```python
from build123d import *

# Parameters (mm, degrees)
BOSS_EXTRUDE1_DEPTH = 10
SKETCH2_W           = 10
SKETCH2_H           = 3
BOSS_EXTRUDE2_DEPTH = 10
SKETCH3_R           = 1.5
CUT_EXTRUDE1_DEPTH  = 3
FILLET1_R           = 15
SKETCH4_R           = 1.5
BOSS_EXTRUDE3_DEPTH = 3
FILLET2_R           = 5


with BuildPart() as part:
    # Sketch1 → Boss-Extrude1 (new body)
    with BuildSketch(Plane.XY):
        Polygon((0, 0), (100, 0), (100, 3), (3, 3), (3, 85), (0, 85), align=None)
    extrude(amount=BOSS_EXTRUDE1_DEPTH)

    # Sketch2 → Boss-Extrude2 (add)
    with BuildSketch(Plane.XY.offset(10)):
        with Locations((95, 1.5)):
            Rectangle(SKETCH2_W, SKETCH2_H)
    extrude(amount=BOSS_EXTRUDE2_DEPTH)

    # Sketch3 → Cut-Extrude1 (cut)
    with BuildSketch(Plane(origin=(0, 3, 0), x_dir=(1, 0, 0), z_dir=(0, 1, 0))):
        with Locations(Location((95, -5, 0), (0, 0, 270))):
            Circle(SKETCH3_R)
        with Locations(Location((95, -15, 0), (0, 0, 90))):
            Circle(SKETCH3_R)
    extrude(amount=-CUT_EXTRUDE1_DEPTH, mode=Mode.SUBTRACT)

    # Fillet1
    fillet1_edges = [part.edges().sort_by_distance(p)[0] for p in [
        (3, 3, 5),
        (0, 0, 5),
    ]]
    fillet(fillet1_edges, radius=FILLET1_R)

    # Sketch4 → Boss-Extrude3 (add)
    with BuildSketch(Plane(origin=(3, 0, 0), x_dir=(0, 0, -1), z_dir=(1, 0, 0))):
        Polygon((0, 100), (-25, 100), (0, 75), align=None)
        with Locations(Location((-12.5, 95.25, 0), (0, 0, 90))):
            Circle(SKETCH4_R, mode=Mode.SUBTRACT)
        with Locations(Location((-4.75, 95.25, 0), (0, 0, 90))):
            Circle(SKETCH4_R, mode=Mode.SUBTRACT)
        with Locations(Location((-4.75, 87.5, 0), (0, 0, 90))):
            Circle(SKETCH4_R, mode=Mode.SUBTRACT)
    extrude(amount=-BOSS_EXTRUDE3_DEPTH)

    # Fillet2
    fillet2_edges = [part.edges().sort_by_distance(p)[0] for p in [
        (1.5, 85, 10),
        (1.5, 100, 25),
    ]]
    fillet(fillet2_edges, radius=FILLET2_R)


solid = part.part
```
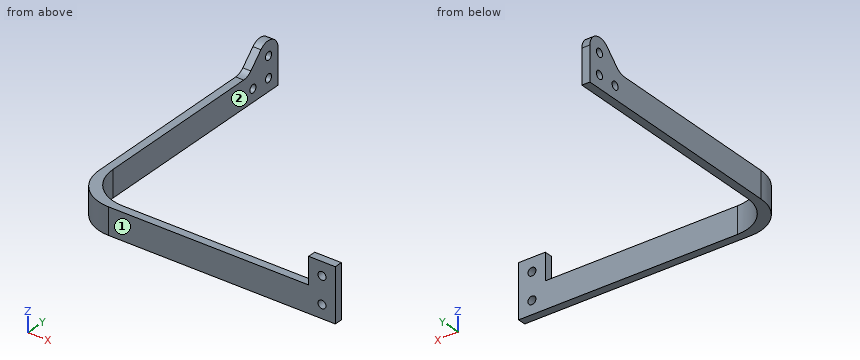
Could you check a few things on this model? Use its own coordinates, in mm. Face numbers are marked on the shaded views. A direction names the side the tool comes from. Round coordinates to 2 decimals unless told otherwise and drop trailing zeros. Write each loop counter-clockwise with the first axis right and the second up, starting at its lowest first coordinate (ties: lowest second). Pieces come first, ordered by that corner, then holes.
(1) For pin 1 (10 mm diameter, centred on x = 48, z = 11, fed in from +Y); pin 2 (2.5 mm diameter, centred on y = 1, z = 14.5, fed in from -X), each with a flat end and sliding along its axis, tell me the tip position at first contact or that it passes through.
Findings below:
pin 1: stops at y = 3
pin 2: stops at x = 90
(2) Suppose I cut it at C-C on y = 62.5. Write out the boundary of the cut face in (x, z).
Findings below:
outline: (0, 0) - (3, 0) - (3, 10) - (0, 10) - close
(3) Suppose I cut it at A-A on x = 95. Write out the boundary of the cut face in (y, z).
Findings below:
outline: (0, 0) - (3, 0) - (3, 3.5) - (0, 3.5) - close; (0, 6.5) - (3, 6.5) - (3, 13.5) - (0, 13.5) - close; (0, 16.5) - (3, 16.5) - (3, 20) - (0, 20) - close
(4) Suppose I cut it at B-B on y = 95.25. Write out the boundary of the cut face in (x, z).
Findings below:
outline: (0, 0) - (3, 0) - (3, 3.25) - (0, 3.25) - close; (0, 6.25) - (3, 6.25) - (3, 11) - (0, 11) - close; (0, 14) - (3, 14) - (3, 17.92) - (0, 17.92) - close
(5) If I drill on probe 1 along Z at (x, y) = (1.75, 95.25); probe 2 along X at (y, z) = (2.35, 15); probe 3 along Z at (x, y) = (95, 2.2), over which ranges is the centre line in solid material (lowest first)?
Findings below:
probe 1: z = 0 to 3.25, 6.25 to 11, 14 to 17.92
probe 2: x = 90 to 93.5, 96.5 to 100
probe 3: z = 0 to 3.5, 6.5 to 13.5, 16.5 to 20
(6) Which directions (+Z, -Z, +X, -X, +Y, -Y) give clear straight access to the entire face, cutting with the end or side of a thin tool? Please do the marked faces 1 and 2.
Findings below:
face 1: +Z, -Z, +X, -X, -Y
face 2: +Z, -Z, +X, +Y
